from build123d import *

# Parameters (mm, degrees)
F0_W     = 70
F0_H     = 50
F1_DEPTH = 55.8
F2_R     = 5
F3_R     = 5
F4_W     = 31.709628962
F4_H     = 40
F5_DEPTH = 25
F6_R     = 5
F7_R     = 8.0311344771
F8_DEPTH = 25


with BuildPart() as f1:
    # F0 (on Top) → F1 (new body)
    with BuildSketch(Plane.XY):
        with Locations((-9.0379202738, -0.8199248582)):
            Rectangle(F0_W, F0_H)
    extrude(amount=F1_DEPTH)

    # F2
    f2_edges = [f1.edges().sort_by_distance(p)[0] for p in [
        (-9.03792, -25.819925, 55.8),
    ]]
    fillet(f2_edges, radius=F2_R)

    # F3
    f3_edges = [f1.edges().sort_by_distance(p)[0] for p in [
        (-9.03792, 24.180075, 55.8),
    ]]
    fillet(f3_edges, radius=F3_R)

    # F4 (on face) → F5 (cut)
    with BuildSketch(Plane.XY.offset(55.8)):
        Polygon((30.625000596, 31.9975502789), (-5.7475492358, 31.9975502789), (-5.7475492358, 19.1800751418), (25.9620797262, 19.1800751418), (25.9620797262, -20.8199248582), (-5.7475492358, -20.8199248582), (-5.7475492358, -34.0563766658), (30.625000596, -34.0563766658), align=None)
        with Locations((10.1072652452, -0.8199248582)):
            Rectangle(F4_W, F4_H)
    extrude(amount=-F5_DEPTH, mode=Mode.SUBTRACT)

    # F6
    f6_edges = [f1.edges().sort_by_distance(p)[0] for p in [
        (10.107265, 24.180075, 30.8),
        (25.96208, -0.819925, 30.8),
        (10.107265, -25.819925, 30.8),
        (-5.747549, -0.819925, 30.8),
        (-5.747549, -0.819925, 55.8),
        (-5.747549, 22.715609, 54.335534),
        (-5.747549, -24.355459, 54.335534),
    ]]
    fillet(f6_edges, radius=F6_R)

    # F7 (on face) → F8 (join)
    with BuildSketch(Plane.YZ.offset(25.9620797262)):
        with Locations((0, 14.312678948)):
            Circle(F7_R)
    extrude(amount=F8_DEPTH)


solid = f1.part
Part model, mm, in its own coordinate system. A direction names the side the tool comes from. Coordinates: 2 decimals unless noted, no trailing zeros. Loops run counter-clockwise (first coordinate to the right, second up) from the corner with the lowest first, then second, coordinate; pieces in that order, holes last. Notation, with made-up numbers: (37.25, 12.5) - (76.25, 12.5) arc R12 cw to (76.25, 26.5) - close; hole circle Ø1 at (36.25, 5.25). An arc over 180 degrees is marked (long way). Write each question's results on one line, items separated by ' | '. Start each with the question number.
Q1. Which spindle directions (+Z, -Z, +X, -X, +Y, -Y) get a long thin tool onto all of the face, cutting with end or side? Do faces 1 (the flat face through (-5.748, -1, 43)), 2 (the cylindrical face through (12.79, 22.75, 29.3)), 3 (the flat face through (50.962, 0, 14)), 4 (the flat face through (-17, -25.82, 19)), 5 (the cylindrical face through (-7.251, -24.394, 43.195)). Say none if no direction does.
Q2. Slice it at D-D on y = 0. Give the cut face in (x, z).
Q3. Drop flat-ended pins along their axis: pin 1 Ø1 at (y, z) = (-5, 29.5) entering from +X; pin 2 Ø12 at (y, z) = (9, 42) entering from +X; pin 3 Ø11 at (x, y) = (13, 7.5) entering from +Z. Give the stop position or say it passes through.
Q4. Slice it at B-B on x = 1. Give the cut face in (y, z).
Q5. Slice it at C-C on z = 41. Give the cut face in (x, y), and give its area (3 significant figures).
Q6. Probe line 1 along X through (y, z) = (15, 9); line 2 along Z through (x, y) = (1.5, -16); line 3 along X through (y, z) = (14.5, 46.5). List the from-to ranges inside material, lowest first.
Q7. Slice it at A-A on y = -10. Give the cut face in (x, z).
Answer:
1) face 1: +Z, +X, +Y, -Y | face 2: +Z, +X, +Y | face 3: +Z, -Z, +X, +Y, -Y | face 4: +Z, -Z, +X, -X, -Y | face 5: +Z, +X, -Y
2) outline: (-44.04, 0) - (25.96, 0) - (25.96, 6.28) - (50.96, 6.28) - (50.96, 22.34) - (25.96, 22.34) - (25.96, 25.8) arc R5 ccw to (20.96, 30.8) - (-0.75, 30.8) arc R5 cw to (-5.75, 35.8) - (-5.75, 50.8) arc R5 ccw to (-10.75, 55.8) - (-44.04, 55.8) - close
3) pin 1: stops at x = 24.8 | pin 2: stops at x = -5.75 | pin 3: stops at z = 30.8
4) outline: (-25.82, 0) - (24.18, 0) - (24.18, 25.8) arc R5 ccw to (19.18, 30.8) - (-20.82, 30.8) arc R5 ccw to (-25.82, 25.8) - close
5) outline: (-44.04, -25.82) - (-10.75, -25.82) arc R5 ccw to (-5.75, -20.82) - (-5.75, 19.18) arc R5 ccw to (-10.75, 24.18) - (-44.04, 24.18) - close | area: 1,900 mm2
6) line 1: x = -44.04 to 25.96 | line 2: z = 0 to 30.8 | line 3: x = -44.04 to -5.75
7) outline: (-44.04, 0) - (25.96, 0) - (25.96, 25.8) arc R5 ccw to (20.96, 30.8) - (-0.75, 30.8) arc R5 cw to (-5.75, 35.8) - (-5.75, 50.8) arc R5 ccw to (-10.75, 55.8) - (-44.04, 55.8) - close
